Here's how the part is built. I have some questions about the finished solid (model axes, mm). A direction names the side the tool comes from. Give positions to 0.01 mm unless a question says otherwise; leave off trailing zeros. Loops run counter-clockwise (first coordinate to the right, second up) from the corner with the lowest first, then second, coordinate; pieces in that order, holes last.
Q1. Suppose I cut it at A-A (x = 0). List the corners of the cut face in (y, z) for me.
Q2. Thinking about a two-plate mould opening in Z: for faces 1 (the face through (3, 0, 0)), 2 (the face through (0, 10, 0)), 3 (the face through (-3, 24.6, -1.8)), which applies, pulls with the +Z half, pulls with the -Z half, needs draft (parallel to the pull), parting line crosses it, or undercut?
Q3. For faces 4 (the face through (-0.338, 5.07, -2.578)), 5 (the face through (0, 40, 0)), 6 (the face through (-3.045, 24.65, 1.726)), which set-ups out of +Z, -Z, +X, -X, +Y, -Y let a thin tool reach every point of the face, with its end or its side?
Q4. Suppose I cut it at D-D (x = 3.5). List the corners of the cut face in (y, z) for me, and give its area (3 significant figures).
Q5. Suppose I cut it at B-B (z = -1.25). List the corners of the cut face in (x, y) for me, and give its area (3 significant figures).
Q6. Suppose I cut it at C-C (y = 28). List the corners of the cut face in (x, z) for me, and give its area (3 significant figures).
Q7. I need wall thicknesses on probe 1 along Z at (x, y) = (0, 45.75); probe 2 along X at (y, z) = (3.75, 0); probe 3 along Y at (x, z) = (0.25, -2). Which ranges of each line are inside material? Lowest first, please.
Q8. I'm going to push flat-ended pins straight in: P1, Ø1.6, axis at x = -0.5, z = -0.5, coming from the -Y side; P2, Ø4, axis at y = 9, z = -2.5, coming from the +X side. Where does each tip first touch, or does it pass through?
```python
from build123d import *

# Parameters (mm, degrees)
EXTRUDE_1_DEPTH     = 50
SKETCH_2_R          = 2.6
CUT_EXTRUDE_1_DEPTH = 51
SKETCH_3_R          = 2.6
EXTRUDE_2_DEPTH     = 30


with BuildPart() as part:
    # 草图1 → 凸台-拉伸1 (new body)
    with BuildSketch(Plane(origin=(0, 0, 0), x_dir=(1, 0, 0), z_dir=(0, 1, 0))):
        Polygon((4.041451884, 0), (2.020725942, 3.5), (-2.020725942, 3.5), (-4.041451884, 0), (-2.020725942, -3.5), (2.020725942, -3.5), align=None)
    extrude(amount=EXTRUDE_1_DEPTH)

    # 草图2 → 切除-拉伸1 (cut, through all)
    with BuildSketch(Plane(origin=(0, 50, 0), x_dir=(1, 0, 0), z_dir=(0, 1, 0))):
        Circle(SKETCH_2_R)
    extrude(amount=-CUT_EXTRUDE_1_DEPTH, mode=Mode.SUBTRACT)

    # 草图3 → 凸台-拉伸2 (add)
    with BuildSketch(Plane(origin=(0, 10, 0), x_dir=(-1, 0, 0), z_dir=(0, -1, 0))):
        Circle(SKETCH_3_R)
    extrude(amount=-EXTRUDE_2_DEPTH)


solid = part.part
```
Solutions:
1. outline: (0, -3.5) - (50, -3.5) - (50, -2.6) - (40, -2.6) - (40, 2.6) - (50, 2.6) - (50, 3.5) - (0, 3.5) - (0, 2.6) - (10, 2.6) - (10, -2.6) - (0, -2.6) - close
2. face 1: needs draft
2. face 2: undercut
2. face 3: pulls with the -Z half
3. face 4: -Y
3. face 5: +Y
3. face 6: +Z, -X, +Y, -Y
4. outline: (0, -0.94) - (50, -0.94) - (50, 0.94) - (0, 0.94) - close
4. area: 93.8 mm2
5. outline: (-3.32, 0) - (-2.28, 0) - (-2.28, 10) - (2.28, 10) - (2.28, 0) - (3.32, 0) - (3.32, 50) - (2.28, 50) - (2.28, 40) - (-2.28, 40) - (-2.28, 50) - (-3.32, 50) - close
5. area: 241 mm2
6. outline: (-4.04, 0) - (-2.02, -3.5) - (2.02, -3.5) - (4.04, 0) - (2.02, 3.5) - (-2.02, 3.5) - close
6. area: 42.4 mm2
7. probe 1: z = -3.5 to -2.6, 2.6 to 3.5
7. probe 2: x = -4.04 to -2.6, 2.6 to 4.04
7. probe 3: y = 10 to 40
8. P1: stops at y = 10
8. P2: stops at x = 3.75
